from build123d import *

# Parameters (mm, degrees)
SKETCH2_R          = 2.5
SKETCH2_R_2        = 7.5
CUT_EXTRUDE1_DEPTH = 50.468424272
FILLET1_R          = 1.5


with BuildPart() as part:
    # Sketch1 → Revolve1 (revolve)
    with BuildSketch(Plane.XY, mode=Mode.PRIVATE) as revolve1_sk:
        Polygon((31.75, -3), (32.75, -3), (32.75, 0), (33.75, 0), (33.75, 10), (0, 10), (0, 6), (31.75, 6), align=None)
    revolve(revolve1_sk.sketch.rotate(Axis((0, 10, 0), (0, -1, 0)), 180), axis=Axis((0, 10, 0), (0, -1, 0)))

    # Sketch2 → Cut-Extrude1 (cut, through all)
    with BuildSketch(Plane(origin=(0, 10, 0), x_dir=(1, 0, 0), z_dir=(0, 1, 0))):
        with Locations(Location((0, -19.75, 0), (0, 0, 180))):
            Circle(SKETCH2_R)
        with Locations(Location((-17.104001725, 9.875, 0), (0, 0, 180))):
            Circle(SKETCH2_R)
        with Locations(Location((17.104001725, 9.875, 0), (0, 0, 180))):
            Circle(SKETCH2_R)
        with Locations(Location((0, 0, 0), (0, 0, 180))):
            Circle(SKETCH2_R_2)
    extrude(amount=-CUT_EXTRUDE1_DEPTH, mode=Mode.SUBTRACT)

    # Fillet1
    fillet1_edges = [part.edges().sort_by_distance(p)[0] for p in [
        (33.75, 10, 0),
    ]]
    fillet(fillet1_edges, radius=FILLET1_R)


solid = part.part
Can you work these out from the model? Positions are in its coordinate system, mm. A direction names the side the tool comes from. Round coordinates to 2 decimals unless told otherwise and drop trailing zeros. Write each loop counter-clockwise with the first axis right and the second up, starting at its lowest first coordinate (ties: lowest second). Pieces come first, ordered by that corner, then holes. Notation, with made-up numbers: (6, 76.5) -> (47, 76.5) arc R10 ccw to (47, 93.5) -> close; hole circle Ø3 at (-3.75, 63). An arc over 180 degrees is marked (long way). Use one line per item in the form item = value. Start each with the question number.
Q1. Imagine slicing it at C-C (y = 4.75). Please give me the cut outline in (x, z), then the cut area to 3 significant figures.
Q2. If I drill on probe 1 along X at (y, z) = (2.25, 1); probe 2 along Y at (x, z) = (6, 12.5); probe 3 along X at (y, z) = (0.75, -8.5), over which ranges is the centre line in solid material (lowest first)? Write a range as [from, to].
Q3. I'm going to push flat-ended pins straight in: P1, Ø5, axis at y = -1.5, z = -2.5, coming from the +X side; P2, Ø4, axis at y = 5, z = -18, coming from the -X side; P3, Ø6, axis at x = -9.5, z = -20, coming from the -Y side; P4, Ø10, axis at x = 22.5, z = 26, coming from the +Y side. Where does each tip first touch, or does it pass through?
Q4. Imagine slicing it at A-A (x = 0). Please give me the cut outline in (y, z).
Q5. Which directions (+Z, -Z, +X, -X, +Y, -Y) give clear straight access to the entire face, cutting with the end or side of a thin tool? Please do faces 4 (the face through (-31.238, -1.479, -9.837)), 5 (the face through (-17, -3, -27)).
Q6. We'd pull the mould along X, two halves only. Please class faces 1 (the face through (6.883, 1.437, 30.995)), 2 (the face through (0, 10, -8)), 3 (the face through (7.316, 4.31, 32.947)): +X half, -X half, draft (parallel to the pull), parting line (faces both ways), or undercut.
Q7. Imagine slicing it at B-B (z = 0). Please give me the cut outline in (x, y), then the cut area to 3 significant figures.
Worked out:
q1.outline = circle Ø67.5 at (0, 0); hole circle Ø63.5 at (0, 0)
q1.area = 412 mm^2
q2.probe_1 = [-33.74, -31.73], [31.73, 33.74]
q2.probe_2 = [6, 10]
q2.probe_3 = [-32.66, -30.59], [30.59, 32.66]
q3.P1 = 33.75
q3.P2 = -29.72
q3.P3 = 6
q3.P4 = 10
q4.outline = (-3, -32.75) -> (0, -32.75) -> (0, -33.75) -> (8.5, -33.75) arc R1.5 ccw to (10, -32.25) -> (10, -7.5) -> (6, -7.5) -> (6, -31.75) -> (-3, -31.75) -> close; (-3, 31.75) -> (6, 31.75) -> (6, 22.25) -> (10, 22.25) -> (10, 32.25) arc R1.5 ccw to (8.5, 33.75) -> (0, 33.75) -> (0, 32.75) -> (-3, 32.75) -> close; (6, 7.5) -> (10, 7.5) -> (10, 17.25) -> (6, 17.25) -> close
q5.face_4 = -Y
q5.face_5 = +Z, -Z, +X, -X, -Y
q6.face_1 = undercut
q6.face_2 = draft
q6.face_3 = parting line
q7.outline = (-33.75, 0) -> (-32.75, 0) -> (-32.75, -3) -> (-31.75, -3) -> (-31.75, 6) -> (-7.5, 6) -> (-7.5, 10) -> (-32.25, 10) arc R1.5 ccw to (-33.75, 8.5) -> close; (7.5, 6) -> (31.75, 6) -> (31.75, -3) -> (32.75, -3) -> (32.75, 0) -> (33.75, 0) -> (33.75, 8.5) arc R1.5 ccw to (32.25, 10) -> (7.5, 10) -> close
q7.area = 239 mm^2
